Answer from the drawing. Dimensions are ordinates in mm from the lowest x, y and z of the part. A direction names the side the tool comes from. Give positions to 0.01 mm unless a question says otherwise; leave off trailing zeros. Order: outer loops, then holes, each group sorted by start corner. A loop starts at its lowest first (then second) coordinate and runs counter-clockwise, first axis right, second up. Notation, with made-up numbers: (16, 34) - (24, 34) arc R19 cw to (24, 46) - close; hole circle Ø8 at (24, 0). An arc over 180 degrees is marked (long way). Answer in a Markdown table with one row per item.
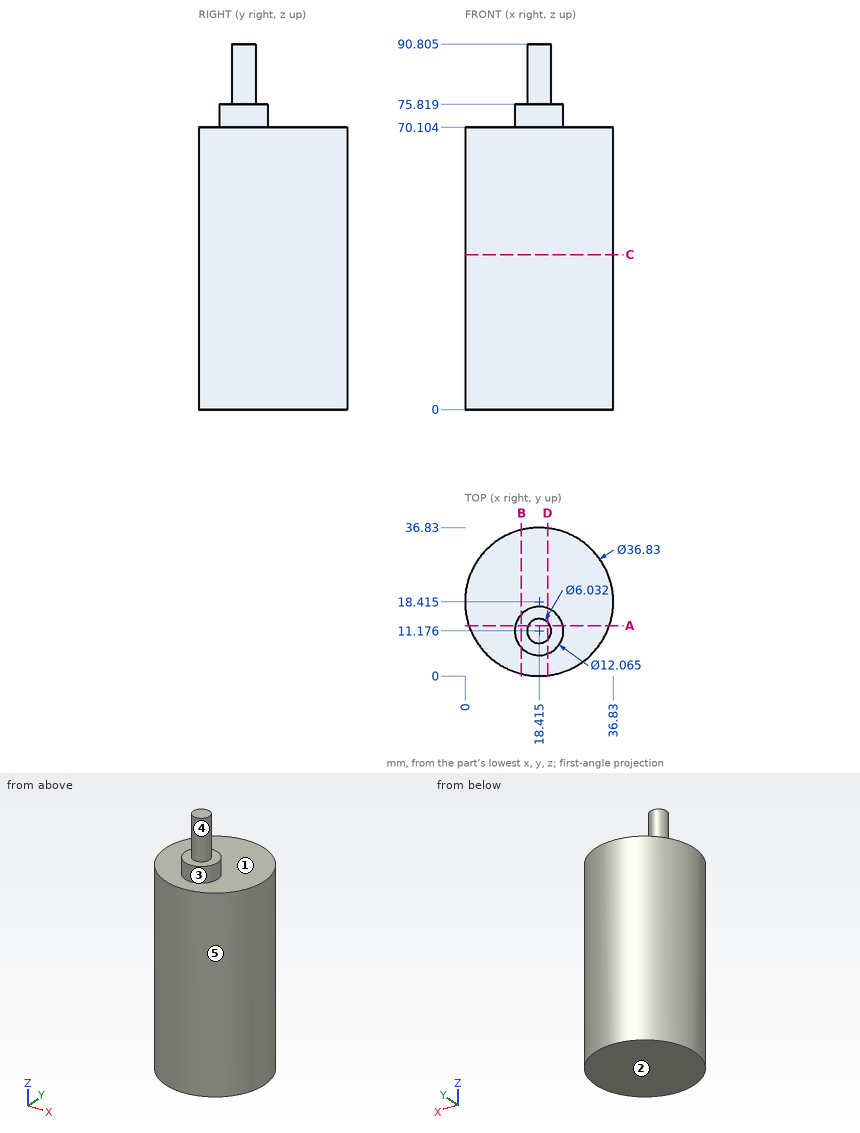
Item 1: Which of the six approach directions +Z, -Z, +X, -X, +Y, -Y give full straight-line access (tool end or side, diameter ignored) to the marked faces 4 and 5?
Answer block:
| item | result |
|---|---|
| face 4 | +Z |
| face 5 | +Z, -Z |
Item 2: Consider line 1 (Z direction, x = 3.5, y = 9.5) (1 decimal); line 2 (Y direction, x = 18, z = 51) (1 decimal); line 3 (Z direction, x = 19.5, y = 6). Determine where each line is inside the solid, lowest interval first.
Answer block:
| item | result |
|---|---|
| line 1 | 0 to 70.1 |
| line 2 | 0 to 36.8 |
| line 3 | 0 to 75.82 |
Item 3: Find section A-A on y = 12.5. Write down the section's boundary in (x, z) (1 decimal).
Answer block:
| item | result |
|---|---|
| outline | (1, 0) - (35.9, 0) - (35.9, 70.1) - (24.3, 70.1) - (24.3, 75.8) - (21.1, 75.8) - (21.1, 90.8) - (15.7, 90.8) - (15.7, 75.8) - (12.5, 75.8) - (12.5, 70.1) - (1, 70.1) - close |
Item 4: Find section D-D on x = 20.5. Write down the section's boundary in (y, z) (1 decimal).
Answer block:
| item | result |
|---|---|
| outline | (0.1, 0) - (36.7, 0) - (36.7, 70.1) - (16.8, 70.1) - (16.8, 75.8) - (13.4, 75.8) - (13.4, 90.8) - (9, 90.8) - (9, 75.8) - (5.5, 75.8) - (5.5, 70.1) - (0.1, 70.1) - close |
Item 5: Determine the mould class of the marked faces 1, 2 and 3 for opening direction Z: pulls with the +Z half, pulls with the -Z half, needs draft (parallel to the pull), parting line crosses it, or undercut.
Answer block:
| item | result |
|---|---|
| face 1 | pulls with the +Z half |
| face 2 | pulls with the -Z half |
| face 3 | needs draft |
Item 6: Find section C-C on z = 38.5. Write down the section's boundary in (x, y) (1 decimal).
Answer block:
| item | result |
|---|---|
| outline | circle Ø36.8 at (18.4, 18.4) |
Item 7: Each of these flat-tipped pins is pushed along its axis until it touches: P1, Ø5, axis at x = 7, z = 30.5, coming from the -Y side; P2, Ø2, axis at x = 22, y = 13.5, coming from the +Z side; P3, Ø8, axis at y = 28, z = 15, coming from the +X side. Where does it stop, or does it pass through?
Answer block:
| item | result |
|---|---|
| P1 | y = 2.3 |
| P2 | z = 75.82 |
| P3 | x = 35.96 |
Item 8: Find section B-B on x = 14. Write down the section's boundary in (y, z) (1 decimal), then the cut area to 3 significant figures.
Answer block:
| item | result |
|---|---|
| outline | (0.5, 0) - (36.3, 0) - (36.3, 70.1) - (15.3, 70.1) - (15.3, 75.8) - (7.1, 75.8) - (7.1, 70.1) - (0.5, 70.1) - close |
| area | 2,550 mm² |
